```python
from build123d import *

# Parameters (mm, degrees)
F0_W     = 609.6
F0_H     = 101.6
F1_DEPTH = 12.7
F2_R     = 38.1
F3_DEPTH = 25.4
F4_DEPTH = 152.4
F5_R     = 38.1
F6_DEPTH = 25.4


with BuildPart() as f1:
    # F0 (on Right) → F1 (new body, symmetric)
    with BuildSketch(Plane.YZ):
        Rectangle(F0_W, F0_H)
    extrude(amount=F1_DEPTH, both=True)

    # F2 (on face) → F3 (cut)
    with BuildSketch(Plane.YZ.offset(12.7)):
        with Locations((-228.6, 0)):
            Circle(F2_R)
        with Locations((228.6, 0)):
            Circle(F2_R)
    extrude(amount=-F3_DEPTH, mode=Mode.SUBTRACT)

    # F4 (add): a face of the model
    f4_faces = [f1.faces().sort_by_distance(p)[0] for p in [
        (0, 304.8, 0),
    ]]
    extrude(f4_faces, amount=F4_DEPTH)

    # F5 (on face) → F6 (cut)
    with BuildSketch(Plane.YZ.offset(12.7)):
        with Locations((381, 0)):
            Circle(F5_R)
    extrude(amount=-F6_DEPTH, mode=Mode.SUBTRACT)


solid = f1.part
```
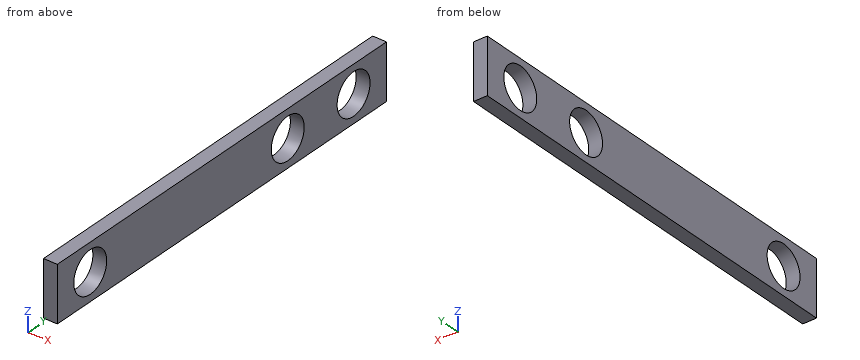
Verification items for the finished model (mm, model axes). Coordinates: 2 decimals unless noted, no trailing zeros. Write each loop counter-clockwise with the first axis right and the second up, starting at its lowest first coordinate (ties: lowest second). Pieces come first, ordered by that corner, then holes. Notation, with made-up numbers: (73, 48.25) - (87, 48.25) arc R9 cw to (87, 55.25) - close; hole circle Ø9 at (-33, -23). An arc over 180 degrees is marked (long way). Write item = value, one per line.
Q1. Cross-section at D-D (z = 27). Enter the section's corners in (x, y).
Answer:
outline = (-12.7, -304.8) - (12.7, -304.8) - (12.7, -255.48) - (-12.7, -255.48) - close; (-12.7, -201.72) - (12.7, -201.72) - (12.7, 201.72) - (-12.7, 201.72) - close; (-12.7, 255.48) - (12.7, 255.48) - (12.7, 354.12) - (-12.7, 354.12) - close; (-12.7, 407.88) - (12.7, 407.88) - (12.7, 457.2) - (-12.7, 457.2) - close
Q2. Material ranges on L1, parallel to Y at x = -1, z = -1.5; L2, parallel to Y at x = -2.75, z = -2; L3, parallel to Z at x = -4.5, y = 381, recorded low to high. Write a range as from..to.
Answer:
L1 = -304.8..-266.67, -190.53..190.53, 266.67..342.93, 419.07..457.2
L2 = -304.8..-266.65, -190.55..190.55, 266.65..342.95, 419.05..457.2
L3 = -50.8..-38.1, 38.1..50.8
Q3. Cross-section at B-B (y = 381). Enter the section's corners in (x, z), plus the area to 3 significant figures.
Answer:
outline = (-12.7, -50.8) - (12.7, -50.8) - (12.7, -38.1) - (-12.7, -38.1) - close; (-12.7, 38.1) - (12.7, 38.1) - (12.7, 50.8) - (-12.7, 50.8) - close
area = 645 mm²
Q4. Cross-section at C-C (x = 1). Enter the section's corners in (y, z).
Answer:
outline = (-304.8, -50.8) - (457.2, -50.8) - (457.2, 50.8) - (-304.8, 50.8) - close; hole circle Ø76.2 at (-228.6, 0); hole circle Ø76.2 at (228.6, 0); hole circle Ø76.2 at (381, 0)
Q5. Cross-section at A-A (z = 0). Enter the section's corners in (x, y).
Answer:
outline = (-12.7, -304.8) - (12.7, -304.8) - (12.7, -266.7) - (-12.7, -266.7) - close; (-12.7, -190.5) - (12.7, -190.5) - (12.7, 190.5) - (-12.7, 190.5) - close; (-12.7, 266.7) - (12.7, 266.7) - (12.7, 342.9) - (-12.7, 342.9) - close; (-12.7, 419.1) - (12.7, 419.1) - (12.7, 457.2) - (-12.7, 457.2) - close
